Geometry: final body of the model. Coordinates: model frame, mm. Round coordinates to 2 decimals unless told otherwise and drop trailing zeros. Order: outer loops, then holes, each group sorted by start corner. A loop starts at its lowest first (then second) coordinate and runs counter-clockwise, first axis right, second up. Notation, with made-up numbers: M 38,71 L 64,71 A21 ccw 64,105 Z; hole C 33.5,-23 d1. An arc over 180 degrees is marked long. Return JSON: item names as keys, results as strings. Group by question number.
Q1. Contact query for flat-ended pins moving along their axis: pin 1 (6 mm diameter, centred on y = -137, z = 7.5, fed in from +X); pin 2 (1 mm diameter, centred on x = -1338.5, z = 12.5, fed in from +Y); pin 3 (12 mm diameter, centred on x = -1420.5, z = 6.5, fed in from -Y). Output: stop coordinate, or through.
Q2. Ray query, probe 1 along Y at (x, z) = (-1570, 15.5); probe 2 along Y at (x, z) = (-1025.5, 1). Return the intervals inside material, ascending.
Q3. Cut plane A-A on z = 4.75. Output: boundary loops of the cut face in (x, y).
Q4. Cut plane B-B on x = -1236. Output: boundary loops of the cut face in (y, z).
```python
from build123d import *

# Parameters (mm, degrees)
F1_DEPTH = 25


with BuildPart() as f1:
    # F0 (on Top) → F1 (new body)
    with BuildSketch(Plane.XY):
        Polygon((0, -360), (0, 0), (-2100, -50), (-2100, -310), align=None)
    extrude(amount=F1_DEPTH)


with BuildPart() as f3:
    # F2 (on face) → F3 (revolve)
    with BuildSketch(Plane.XY.offset(25)):
        Polygon((0, 0), (0, -360), (32.8437872231, -908.5312581062), (103.8437858224, -1328.6146020889), (234.0103685856, -1328.6146020889), (193.9810067415, 1467.5388336182), (68.257547915, 1411.1691713333), (-87.2723832726, 1199.2609500885), (-128.0860751867, 896.1502313614), (-80.0736993551, 367.2015070915), align=None)
    revolve(axis=Axis((213.9956876636, 69.4621157646, 25), (-0.0143144007, 0.9998975437, 0)))


solid = f1.part
```
Result sheet:
{
 "1": {"pin 1": "stops at x = 0", "pin 2": "stops at y = -31.86", "pin 3": "stops at y = -326.32"},
 "2": {"probe 1": "y = -322.62 to -37.38", "probe 2": "y = -335.58 to -24.42"},
 "3": {"outline": "M -2100,-310 L 0,-360 L 0,0 L -2100,-50 Z"},
 "4": {"outline": "M -330.57,0 L -29.43,0 L -29.43,25 L -330.57,25 Z"}
}
